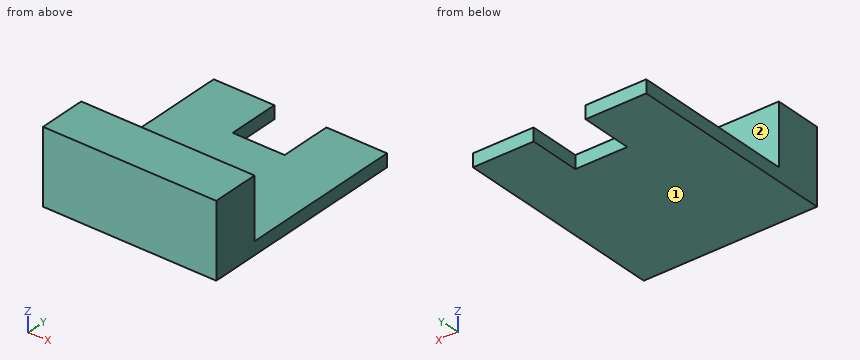
from build123d import *

# Parameters (mm, degrees)
F0_W     = 55
F0_H     = 70
F1_DEPTH = 100
F2_W     = 200
F2_H     = 190.7
F2_H_2   = 55
F3_DEPTH = 15
F4_W     = 60
F4_H     = 60
F5_DEPTH = 25


with BuildPart() as f1:
    # F0 (on Right) → F1 (new body, symmetric)
    with BuildSketch(Plane.YZ):
        Rectangle(F0_W, F0_H)
    extrude(amount=F1_DEPTH, both=True)

    # F2 (on face) → F3 (join)
    with BuildSketch(Plane(origin=(0, 0, -35), x_dir=(1, 0, 0), z_dir=(0, 0, -1))):
        with Locations((0, -122.85)):
            Rectangle(F2_W, F2_H)
        Rectangle(F2_W, F2_H_2)
    extrude(amount=F3_DEPTH)

    # F4 (on face) → F5 (cut)
    with BuildSketch(Plane.XY.offset(-35)):
        with Locations((0, 188.2)):
            Rectangle(F4_W, F4_H)
    extrude(amount=-F5_DEPTH, mode=Mode.SUBTRACT)


solid = f1.part
Here's how the part is built. I have some questions about the finished solid (model axes, mm). Face numbers are marked on the shaded views. A direction names the side the tool comes from. Round coordinates to 2 decimals unless told otherwise and drop trailing zeros. Loops run counter-clockwise (first coordinate to the right, second up) from the corner with the lowest first, then second, coordinate; pieces in that order, holes last.
1. If we section it at A-A on z = -44: Write out the boundary of the cut face in (x, y), plus the area to 3 significant figures.
Answer list:
outline: (-100, -27.5) - (100, -27.5) - (100, 218.2) - (30, 218.2) - (30, 158.2) - (-30, 158.2) - (-30, 218.2) - (-100, 218.2) - close
area: 45,500 mm2
2. For P1, Ø2, axis at x = -47.5, z = 11.5, coming from the +Y side; P2, Ø4.5, axis at x = 1, z = -40.5, coming from the +Y side, each with a flat end and sliding along its axis, tell me the tip position at first contact or that it passes through.
Answer list:
P1: stops at y = 27.5
P2: stops at y = 158.2
3. If we section it at D-D on x = 56: Write out the boundary of the cut face in (y, z), plus the area to 3 significant figures.
Answer list:
outline: (-27.5, -50) - (218.2, -50) - (218.2, -35) - (27.5, -35) - (27.5, 35) - (-27.5, 35) - close
area: 7,540 mm2
4. Which directions (+Z, -Z, +X, -X, +Y, -Y) give clear straight access to the entire face, cutting with the end or side of a thin tool? Please do the marked faces 1 and 2.
Answer list:
face 1: -Z, +X, -X, +Y, -Y
face 2: +Z, +X, -X, +Y
5. If we section it at B-B on x = -25.5: Write out the boundary of the cut face in (y, z).
Answer list:
outline: (-27.5, -50) - (158.2, -50) - (158.2, -35) - (27.5, -35) - (27.5, 35) - (-27.5, 35) - close
6. If we section it at C-C on y = 65: Write out the boundary of the cut face in (x, z), plus the area to 3 significant figures.
Answer list:
outline: (-100, -50) - (100, -50) - (100, -35) - (-100, -35) - close
area: 3,000 mm2
7. If I drill on line 1 along Y through (x, z) = (83, -28); line 2 along Z through (x, y) = (18.5, 45.5), over which ranges is the centre line in solid material (lowest first)?
Answer list:
line 1: y = -27.5 to 27.5
line 2: z = -50 to -35
